Source: CAD feature listing. Evaluate the final solid. Frame: model axes, mm. Face numbers are marked on the shaded views. Give positions to 0.01 mm unless a question says otherwise; leave off trailing zeros. Order: outer loops, then holes, each group sorted by start corner. A loop starts at its lowest first (then second) coordinate and runs counter-clockwise, first axis right, second up.
```python
from build123d import *

# Parameters (mm, degrees)
F1_DEPTH = 6.35
F2_R     = 3.175
F3_DEPTH = 12.7
F4_R     = 6.4822420389
F5_DEPTH = 6.35


with BuildPart() as f1:
    # F0 (on Top) → F1 (new body)
    with BuildSketch(Plane.XY):
        with BuildLine():
            Line((0, -17.430102046), (0, 0))
            Line((0, 0), (0, 3.216402))
            ThreePointArc((0, 3.216402), (-6.7351920908, 6.0062099092), (-9.525, 12.741402))
            Line((-9.525, 12.741402), (-9.525, -26.955102046))
            ThreePointArc((-9.525, -26.955102046), (-6.7351920908, -20.2199099552), (0, -17.430102046))
        make_face()
        with BuildLine():
            ThreePointArc((-9.525, 12.741402), (-6.7351920908, 6.0062099092), (0, 3.216402))
            Line((0, 3.216402), (0, 9.566402))
            ThreePointArc((0, 9.566402), (-3.175, 12.741402), (0, 15.916402))
            Line((0, 15.916402), (0, 22.266402))
            ThreePointArc((0, 22.266402), (-6.7351920908, 19.4765940908), (-9.525, 12.741402))
        make_face()
        with BuildLine():
            Line((0, -23.780102046), (0, -17.430102046))
            ThreePointArc((0, -17.430102046), (-6.7351920908, -20.2199099552), (-9.525, -26.955102046))
            ThreePointArc((-9.525, -26.955102046), (-6.7351920908, -33.6902941368), (0, -36.480102046))
            Line((0, -36.480102046), (7.5123847033, -32.8108429103))
            ThreePointArc((7.5123847033, -32.8108429103), (9.007804652, -30.0510801387), (9.525, -26.955102046))
            ThreePointArc((9.525, -26.955102046), (9.2802728088, -24.809837122), (8.5586668568, -22.7748093967))
            Line((8.5586668568, -22.7748093967), (2.8528889523, -25.5616711629))
            ThreePointArc((2.8528889523, -25.5616711629), (3.0934242696, -26.240013738), (3.175, -26.955102046))
            ThreePointArc((3.175, -26.955102046), (-2.2450640303, -29.2001660763), (0, -23.780102046))
        make_face()
        with BuildLine():
            ThreePointArc((9.525, 12.741402), (9.463768469, 11.6631110537), (9.2808611307, 10.5986837096))
            Line((9.2808611307, 10.5986837096), (45.9066000969, 2.1427182904))
            ThreePointArc((45.9066000969, 2.1427182904), (49.2580332078, 7.4543617002), (55.1874612276, 9.525))
            Line((55.1874612276, 9.525), (55.1874612276, 9.7662775009))
            Line((55.1874612276, 9.7662775009), (4.1043156247, 21.3367622748))
            ThreePointArc((4.1043156247, 21.3367622748), (8.0566503997, 17.8223477129), (9.525, 12.741402))
        make_face()
        with BuildLine():
            Line((3.0936203769, 12.0271625699), (9.2808611307, 10.5986837096))
            ThreePointArc((9.2808611307, 10.5986837096), (9.463768469, 11.6631110537), (9.525, 12.741402))
            ThreePointArc((9.525, 12.741402), (8.0566503997, 17.8223477129), (4.1043156247, 21.3367622748))
            Line((4.1043156247, 21.3367622748), (0, 22.266402))
            Line((0, 22.266402), (0, 15.916402))
            ThreePointArc((0, 15.916402), (2.2450640303, 14.9864660303), (3.175, 12.741402))
            ThreePointArc((3.175, 12.741402), (3.1545894897, 12.3819716846), (3.0936203769, 12.0271625699))
        make_face()
        with BuildLine():
            ThreePointArc((55.1874612276, 9.525), (49.2580332078, 7.4543617002), (45.9066000969, 2.1427182904))
            Line((45.9066000969, 2.1427182904), (52.0938408507, 0.7142394301))
            ThreePointArc((52.0938408507, 0.7142394301), (53.210985221, 2.4847872334), (55.1874612276, 3.175))
            Line((55.1874612276, 3.175), (55.1874612276, 9.525))
        make_face()
        with BuildLine():
            ThreePointArc((55.1874612276, -9.525), (50.1422487685, -8.0790752096), (46.6287943708, -4.1802926493))
            Line((46.6287943708, -4.1802926493), (8.5586668568, -22.7748093967))
            ThreePointArc((8.5586668568, -22.7748093967), (9.2802728088, -24.809837122), (9.525, -26.955102046))
            ThreePointArc((9.525, -26.955102046), (9.007804652, -30.0510801387), (7.5123847033, -32.8108429103))
            Line((7.5123847033, -32.8108429103), (55.1874612276, -9.525))
        make_face()
        with BuildLine():
            Line((52.3345722753, -1.3934308831), (46.6287943708, -4.1802926493))
            ThreePointArc((46.6287943708, -4.1802926493), (50.1422487685, -8.0790752096), (55.1874612276, -9.525))
            ThreePointArc((55.1874612276, -9.525), (61.9226533184, -6.7351920908), (64.7124612276, 0))
            ThreePointArc((64.7124612276, 0), (61.9226533184, 6.7351920908), (55.1874612276, 9.525))
            Line((55.1874612276, 9.525), (55.1874612276, 3.175))
            ThreePointArc((55.1874612276, 3.175), (57.4325252579, 2.2450640303), (58.3624612276, 0))
            ThreePointArc((58.3624612276, 0), (55.9025495356, -3.0934242696), (52.3345722753, -1.3934308831))
        make_face()
        with BuildLine():
            ThreePointArc((4.1043156247, 21.3367622748), (2.1041409628, 22.0310852997), (0, 22.266402))
            Line((0, 22.266402), (4.1043156247, 21.3367622748))
        make_face()
        with BuildLine():
            Line((7.5123847033, -32.8108429103), (0, -36.480102046))
            ThreePointArc((0, -36.480102046), (4.1802926493, -35.5137689028), (7.5123847033, -32.8108429103))
        make_face()
        with BuildLine():
            Line((0, 3.216402), (0, 0))
            Line((0, 0), (45.6624612276, 0))
            ThreePointArc((45.6624612276, 0), (45.7236927586, 1.0782909463), (45.9066000969, 2.1427182904))
            Line((45.9066000969, 2.1427182904), (9.2808611307, 10.5986837096))
            ThreePointArc((9.2808611307, 10.5986837096), (5.9294280198, 5.2870402998), (0, 3.216402))
        make_face()
        with BuildLine():
            Line((0, 9.566402), (0, 3.216402))
            ThreePointArc((0, 3.216402), (5.9294280198, 5.2870402998), (9.2808611307, 10.5986837096))
            Line((9.2808611307, 10.5986837096), (3.0936203769, 12.0271625699))
            ThreePointArc((3.0936203769, 12.0271625699), (1.9764760066, 10.2566147666), (0, 9.566402))
        make_face()
        with BuildLine():
            Line((45.6624612276, 0), (0, 0))
            Line((0, 0), (0, -17.430102046))
            ThreePointArc((0, -17.430102046), (5.0452124591, -18.8760268364), (8.5586668568, -22.7748093967))
            Line((8.5586668568, -22.7748093967), (46.6287943708, -4.1802926493))
            ThreePointArc((46.6287943708, -4.1802926493), (45.9071884188, -2.145264924), (45.6624612276, 0))
        make_face()
        with BuildLine():
            ThreePointArc((8.5586668568, -22.7748093967), (5.0452124591, -18.8760268364), (0, -17.430102046))
            Line((0, -17.430102046), (0, -23.780102046))
            ThreePointArc((0, -23.780102046), (1.6817374864, -24.2620769761), (2.8528889523, -25.5616711629))
            Line((2.8528889523, -25.5616711629), (8.5586668568, -22.7748093967))
        make_face()
        with BuildLine():
            Line((52.0124612276, 0), (45.6624612276, 0))
            ThreePointArc((45.6624612276, 0), (45.9071884188, -2.145264924), (46.6287943708, -4.1802926493))
            Line((46.6287943708, -4.1802926493), (52.3345722753, -1.3934308831))
            ThreePointArc((52.3345722753, -1.3934308831), (52.094036958, -0.715088308), (52.0124612276, 0))
        make_face()
        with BuildLine():
            ThreePointArc((45.9066000969, 2.1427182904), (45.7236927586, 1.0782909463), (45.6624612276, 0))
            Line((45.6624612276, 0), (52.0124612276, 0))
            ThreePointArc((52.0124612276, 0), (52.0328717379, 0.3594303154), (52.0938408507, 0.7142394301))
            Line((52.0938408507, 0.7142394301), (45.9066000969, 2.1427182904))
        make_face()
    extrude(amount=F1_DEPTH)

    # F2 (on face) → F3 (join)
    with BuildSketch(Plane.XY.offset(6.35)):
        with BuildLine():
            Line((-9.525, 41.1111302674), (-9.525, 12.741402))
            ThreePointArc((-9.525, 12.741402), (-5.0809457129, 20.7980523997), (4.1043156247, 21.3367622748))
            Line((4.1043156247, 21.3367622748), (12.3195811982, 19.4759801301))
            Line((12.3195811982, 19.4759801301), (5.7150009088, 41.1111302674))
            Line((5.7150009088, 41.1111302674), (-9.525, 41.1111302674))
        make_face()
        with Locations((-0.0769013266, 32.6290909023)):
            Circle(F2_R, mode=Mode.SUBTRACT)
    extrude(amount=-F3_DEPTH)

    # F4 (on face) → F5 (cut)
    with BuildSketch(Plane(origin=(0, 0, -6.35), x_dir=(1, 0, 0), z_dir=(0, 0, -1))):
        with BuildLine():
            Line((-9.525, -41.1111302674), (5.7150009088, -41.1111302674))
            Line((5.7150009088, -41.1111302674), (12.3195811982, -19.4759801301))
            Line((12.3195811982, -19.4759801301), (4.1043156247, -21.3367622748))
            ThreePointArc((4.1043156247, -21.3367622748), (-5.0809457129, -20.7980523997), (-9.525, -12.741402))
            Line((-9.525, -12.741402), (-9.525, -41.1111302674))
        make_face()
        with Locations((-0.0769013266, -32.6290909023)):
            Circle(F4_R, mode=Mode.SUBTRACT)
    extrude(amount=-F5_DEPTH, mode=Mode.SUBTRACT)


solid = f1.part
```
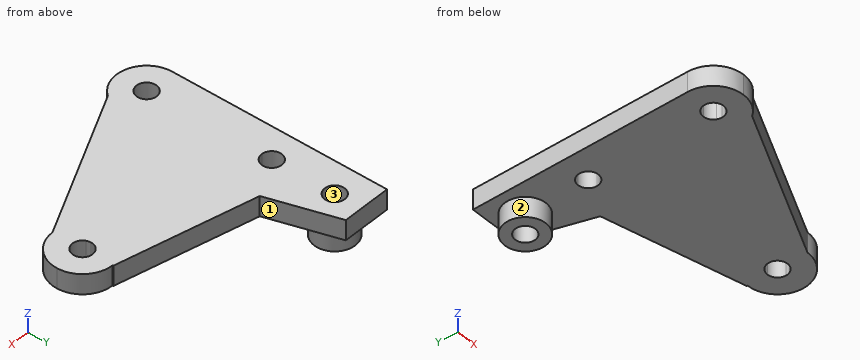
1) Section query D-D, the plane z = -2.5. Return the cut outline in (x, y) (3 decimals), and give its area (3 significant figures).
Report:
outline: circle Ø12.964 at (-0.077, 32.629); hole circle Ø6.35 at (-0.077, 32.629)
area: 100 mm2
2) Section query A-A, the plane x = 1.5. Return the cut outline in (y, z), and give its area (3 significant figures).
Report:
outline: (-36.36, 0) - (-29.75, 0) - (-29.75, 6.35) - (-36.36, 6.35) - close; (-24.16, 0) - (9.94, 0) - (9.94, 6.35) - (-24.16, 6.35) - close; (15.54, 0) - (26.34, 0) - (26.34, -6.35) - (29.87, -6.35) - (29.87, 6.35) - (15.54, 6.35) - close; (35.38, -6.35) - (38.92, -6.35) - (38.92, 0) - (41.11, 0) - (41.11, 6.35) - (35.38, 6.35) - close
area: 431 mm2
3) Material intervals for L1, parallel to Y at x = 1.5, z = 5; L2, parallel to X at y = -19, z = 4.5 (1 decimal); L3, parallel to Z at x = 24.5, y = -4, sorted ascending.
Report:
L1: y = -36.36 to -29.75, -24.16 to 9.94, 15.54 to 29.87, 35.38 to 41.11
L2: x = -9.5 to 35.8
L3: z = 0 to 6.35
4) Pin query (flat end, axial travel): pin 1 (1 mm diameter, centred on x = 13, z = 2.5, fed in from +Y); pin 2 (4 mm diameter, centred on y = 6.5, z = 3.5, fed in from +X); pin 3 (2 mm diameter, centred on x = 54.5, z = 1, fed in from -Y). Return the tip coordinate at first contact, or that it passes through.
Report:
pin 1: stops at y = 19.44
pin 2: stops at x = 63.58
pin 3: stops at y = -10.35
5) Section query C-C, the plane x = 50. Return the cut outline in (y, z).
Report:
outline: (-12.06, 0) - (10.94, 0) - (10.94, 6.35) - (-12.06, 6.35) - close
6) Section query B-B, the plane z = 3. Return the cut outline in (x, y) (3 decimals).
Report:
outline: (-9.525, -26.955) arc R9.525 ccw to (7.512, -32.811) - (55.187, -9.525) arc R9.525 ccw to (55.187, 9.525) - (55.187, 9.766) - (12.32, 19.476) - (5.715, 41.111) - (-9.525, 41.111) - close; hole circle Ø6.35 at (-0.077, 32.629); hole circle Ø6.35 at (0, -26.955); hole circle Ø6.35 at (0, 12.741); hole circle Ø6.35 at (55.187, 0)
7) Draft query along Y for the marked faces 1, 2 and 3. Return one class per face: +Y half, -Y half, draft (parallel to the pull), parting line (faces both ways), or undercut.
Report:
face 1: +Y half
face 2: parting line
face 3: undercut
